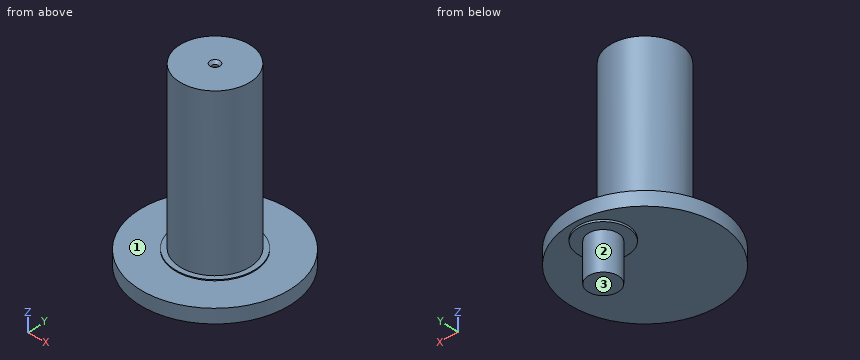
```python
from build123d import *

# Parameters (mm, degrees)
SKETCH1_R                                       = 15
BOSS_EXTRUDE1_DEPTH                             = 2.8
SKETCH3_R                                       = 8
BOSS_EXTRUDE3_DEPTH                             = 0.2
SKETCH2_R                                       = 7
BOSS_EXTRUDE2_DEPTH                             = 33
SKETCH4_R                                       = 5
BOSS_EXTRUDE4_DEPTH                             = 0.4
SKETCH5_R                                       = 3
BOSS_EXTRUDE5_DEPTH                             = 8
CSK_FOR_M2_OVAL_HEAD_MACHINE_SCREW1_D           = 1
CSK_FOR_M2_OVAL_HEAD_MACHINE_SCREW1_DEPTH       = 1
CSK_FOR_M2_OVAL_HEAD_MACHINE_SCREW1_CSINK_D     = 2
CSK_FOR_M2_OVAL_HEAD_MACHINE_SCREW1_CSINK_ANGLE = 90
CSK_FOR_M2_OVAL_HEAD_MACHINE_SCREW1_TIP         = 0.30043031


with BuildPart() as part:
    # Sketch1 → Boss-Extrude1 (new body)
    with BuildSketch(Plane.XY):
        Circle(SKETCH1_R)
    extrude(amount=BOSS_EXTRUDE1_DEPTH)

    # Sketch3 → Boss-Extrude3 (add)
    with BuildSketch(Plane.XY.offset(2.8)):
        Circle(SKETCH3_R)
    extrude(amount=BOSS_EXTRUDE3_DEPTH)

    # Sketch2 → Boss-Extrude2 (add)
    with BuildSketch(Plane.XY.offset(3)):
        Circle(SKETCH2_R)
    extrude(amount=BOSS_EXTRUDE2_DEPTH)

    # Sketch4 → Boss-Extrude4 (add)
    with BuildSketch(Plane(origin=(0, 0, 0), x_dir=(-1, 0, 0), z_dir=(0, 0, -1))):
        with Locations(Location((0, 9, 0), (0, 0, 180))):  # turned: the seam where the file's is
            Circle(SKETCH4_R)
    extrude(amount=BOSS_EXTRUDE4_DEPTH)

    # Sketch5 → Boss-Extrude5 (add)
    with BuildSketch(Plane(origin=(0, 0, 0), x_dir=(-1, 0, 0), z_dir=(0, 0, -1))):
        with Locations((0, 9)):
            Circle(SKETCH5_R)
    extrude(amount=BOSS_EXTRUDE5_DEPTH)

    # CSK for M2 Oval Head Machine Screw1
    with Locations(Plane.XY.offset(36)):
        with Locations((0, 0)):
            CounterSinkHole(CSK_FOR_M2_OVAL_HEAD_MACHINE_SCREW1_D / 2, CSK_FOR_M2_OVAL_HEAD_MACHINE_SCREW1_CSINK_D / 2, depth=CSK_FOR_M2_OVAL_HEAD_MACHINE_SCREW1_DEPTH, counter_sink_angle=CSK_FOR_M2_OVAL_HEAD_MACHINE_SCREW1_CSINK_ANGLE)
            with Locations((0, 0, -(CSK_FOR_M2_OVAL_HEAD_MACHINE_SCREW1_DEPTH + CSK_FOR_M2_OVAL_HEAD_MACHINE_SCREW1_TIP / 2))):  # 118° drill point
                Cone(0, CSK_FOR_M2_OVAL_HEAD_MACHINE_SCREW1_D / 2, CSK_FOR_M2_OVAL_HEAD_MACHINE_SCREW1_TIP, mode=Mode.SUBTRACT)


solid = part.part
```
Check sheet for the modelled part. Datum: model origin and axes. Units: mm. Face numbers are marked on the shaded views. A direction names the side the tool comes from. Give positions to 0.01 mm unless a question says otherwise; leave off trailing zeros. Loops run counter-clockwise (first coordinate to the right, second up) from the corner with the lowest first, then second, coordinate; pieces in that order, holes last. Notation, with made-up numbers: M 85.25,-19.5 L 92.25,-19.5 A8 ccw 92.25,-8.5 Z; hole C -35,53 d3. An arc over 180 degrees is marked long. Answer in a Markdown table with one row per item.
1) Thickness scan on line 1 (Y direction, x = 0, z = 35.35); line 2 (Z direction, x = -1, y = -5); line 3 (Z direction, x = -0.25, y = -8.5). Record the ranges inside material, lowest first.
Solutions:
| item | result |
|---|---|
| line 1 | y = -7 to -0.5, 0.5 to 7 |
| line 2 | z = 0 to 36 |
| line 3 | z = 0 to 2.8 |
2) Cross-section at D-D (y = 13.25). Enter the section's corners in (x, z).
Solutions:
| item | result |
|---|---|
| outline | M -7.03,0 L -2.63,0 L -2.63,-0.4 L 2.63,-0.4 L 2.63,0 L 7.03,0 L 7.03,2.8 L -7.03,2.8 Z |
3) Cross-section at A-A (y = 9). Enter the section's corners in (x, z), plus the area to 3 significant figures.
Solutions:
| item | result |
|---|---|
| outline | M -12,0 L -5,0 L -5,-0.4 L -3,-0.4 L -3,-8 L 3,-8 L 3,-0.4 L 5,-0.4 L 5,0 L 12,0 L 12,2.8 L -12,2.8 Z |
| area | 117 mm^2 |
4) Cross-section at C-C (z = 31). Enter the section's corners in (x, y).
Solutions:
| item | result |
|---|---|
| outline | C 0,0 d14 |
5) Cross-section at B-B (x = 12). Enter the section's corners in (y, z), plus the area to 3 significant figures.
Solutions:
| item | result |
|---|---|
| outline | M -9,0 L 9,0 L 9,2.8 L -9,2.8 Z |
| area | 50.4 mm^2 |
6) Tool access check on the marked faces 1, 2 and 3. Record the directions out of +Z, -Z, +X, -X, +Y, -Y that give a thin tool (end or side, any length) a straight path to the whole face; none if there is none.
Solutions:
| item | result |
|---|---|
| face 1 | +Z |
| face 2 | -Z |
| face 3 | -Z, +X, -X, +Y, -Y |
7) Depth check by flat-ended pin: pin 1 (1 mm diameter, centred on y = -8.5, z = 22.5, fed in from -X); pin 2 (15 mm diameter, centred on x = 2, y = 7, fed in from +Z); pin 3 (4 mm diameter, centred on x = -5.5, z = 17, fed in from -Y); pin 4 (12 mm diameter, centred on x = -11.5, z = 15.5, fed in from +Y). Enter the tip coordinate at first touch or a pass-through.
Solutions:
| item | result |
|---|---|
| pin 1 | passes through |
| pin 2 | stops at z = 36 |
| pin 3 | stops at y = -6.06 |
| pin 4 | stops at y = 4.33 |
